```python
from build123d import *
from build123d import SkipClean  # not in build123d's __all__

# Parameters (mm, degrees)
F2_R          = 5
F3_R          = 2
F4_DEPTH      = 25
F4_DEPTH_BACK = 25
F6_R          = 2


with BuildPart() as f1:
    # F0 (on Front) → F1 (revolve)
    with BuildSketch(Plane.XZ):
        with BuildLine():
            Line((-60, 0), (0, 0))
            ThreePointArc((0, 0), (-7.7499262393, 9.7435706018), (-18.9874336143, 4.3847505093))
            ThreePointArc((-18.9874336143, 4.3847505093), (-31.9220569404, 6.4479089357), (-44.3965084851, 10.4415491223))
            Line((-44.3965084851, 10.4415491223), (-44.3965084851, 13.1515692919))
            Line((-44.3965084851, 13.1515692919), (-48.2224225998, 13.1515692919))
            Line((-48.2224225998, 13.1515692919), (-48.2224225998, 15.8615894616))
            ThreePointArc((-48.2224225998, 15.8615894616), (-52.9723552194, 17.427920622), (-55, 22))
            Line((-55, 22), (-55, 24))
            Line((-55, 24), (-60, 24))
            Line((-60, 24), (-60, 0))
        make_face()
    revolve(axis=Axis((-30, 0, 0), (-1, 0, 0)))

    # F2
    f2_edges = [f1.edges().sort_by_distance(p)[0] for p in [
        (-18.987434, 0, -4.384751),
    ]]
    fillet(f2_edges, radius=F2_R)

    # F3 (on Top) → F4 (cut, two sides)
    with BuildSketch(Plane.XY) as f4_sk:
        with Locations((-10, 0)):
            Circle(F3_R)
    extrude(amount=-F4_DEPTH, mode=Mode.SUBTRACT)
    extrude(f4_sk.sketch, amount=F4_DEPTH_BACK, mode=Mode.SUBTRACT)

    # F7: sweep along a path in F5
    with BuildLine(Plane.XZ) as f7_path:
        Line((-10, 0), (-10, -18.9135132155))
        ThreePointArc((-10, -18.9135132155), (-10.3850895053, -20.8377276333), (-11.4810404502, -22.4655441398))
        Line((-11.4810404502, -22.4655441398), (-18.572177738, -29.4906590134))
    # F6 (on Top) → F7 (sweep)
    with BuildSketch(Plane.XY):
        with Locations((-10, 0)):
            Circle(F6_R)
    sweep(path=f7_path.line)

    # F8: F1 across plane


with BuildPart() as f1_1:
    add(f1.part, clean=False)
    with SkipClean():  # cleaning this boolean's faces spoils the solid; the shape is the same uncleaned
        add(f1.part.mirror(Plane.XY), clean=False)


solid = f1_1.part
```
Model file for the job. Use its own axes, mm. A direction names the side the tool comes from. Round coordinates to 2 decimals unless told otherwise and drop trailing zeros. Write each loop counter-clockwise with the first axis right and the second up, starting at its lowest first coordinate (ties: lowest second). Pieces come first, ordered by that corner, then holes. Notation, with made-up numbers: (-39.5, -1.5) - (15.5, -1.5) arc R34 ccw to (15.5, 31.5) - close; hole circle Ø5 at (65, -14.75). An arc over 180 degrees is marked (long way). Use CSV: the item, a comma, the result in double quotes. Start each with the question number.
Item 1: Pin check, flat tips, straight feed: P1, Ø1, axis at x = -25.5, z = 0.5, coming from the -Y side; P2, Ø10, axis at x = -53, z = -1, coming from the -Y side; P3, Ø10, axis at y = 11.5, z = -5, coming from the +X side. Stop position of each tip, or through.
Item 2: Band-saw the part on B-B (x = -30). Write the cut outline in (y, z), and give its area (3 significant figures).
Item 3: Tool access for faces 1 (the face through (-60, 0, 0)), 2 (the face through (-11.6, 1.2, 14.4)): list every direction of +Z, -Z, +X, -X, +Y, -Y with a clear straight run to the whole face (end or side of a thin tool).
Item 4: Drill centre lines: L1, parallel to X at y = -13.5, z = 17; L2, parallel to X at y = -5, z = -7; L3, parallel to Y at x = -39, z = 4. Where is each one in solid material? Low to high. Write a range as [from, to].
Item 5: Two-plate mould, pull along Z, no slides. Class faces 3 (the face through (-18.552, -0.028, -29.511)), 4 (the face through (-57.535, 1.055, -23.977)), 5 (the face through (-14.427, 1.774, 26.683)): released by +Z, released by -Z, zero draft, split by the parting line, or undercut.
Item 6: Band-saw the part on A-A (x = -46). Write the cut outline in (y, z), and give its area (3 significant figures).
Checked values:
1,P1,"stops at y = -5.24"
1,P2,"stops at y = -24"
1,P3,"stops at x = -3.43"
2,outline,"circle Ø12.03 at (0, 0)"
2,area,"114 mm²"
3,face 1,"+Z, -Z, -X, +Y, -Y"
3,face 2,"none"
4,L1,"x = [-60, -54.99]"
4,L2,"x = [-60, -39.44], [-15.1, -4.9]"
4,L3,"y = [-7.45, 7.45]"
5,face 3,"released by -Z"
5,face 4,"split by the parting line"
5,face 5,"undercut"
6,outline,"circle Ø26.3 at (0, 0)"
6,area,"543 mm²"
